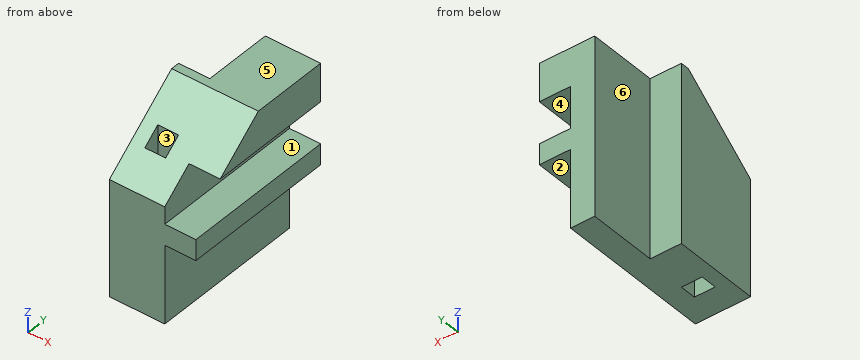
Solid Edge part; units mm, degrees
sketch "Sketch1" plane through (0, 0, 0) normal (0, 0, 1) x (1, 0, 0)
  line L0 (25, -45) -> (25, 45)
  line L1 (25, 45) -> (-25, 45)
  line L2 (-25, 45) -> (-25, -45)
  line L3 (-25, -45) -> (25, -45)
extrude "Protrusion1" add sketch "Sketch1" along normal blind 103
sketch "Sketch2" plane through (0, -45, 51.5) normal (0, -1, 0) x (1, 0, 0)
  line L0 (25, 5.5) -> (25, 29.5)
  line L1 (25, 29.5) -> (7, 29.5)
  line L2 (7, 29.5) -> (7, 5.5)
  line L3 (7, 5.5) -> (25, 5.5)
  line L4 (25, -6.5) -> (25, -51.5)
  line L5 (25, -51.5) -> (7, -51.5)
  line L6 (7, -51.5) -> (7, -6.5)
  line L7 (7, -6.5) -> (25, -6.5)
extrude "Cutout1" cut sketch "Sketch2" against normal up to next
sketch "Sketch3" plane through (-25, 0, 51.5) normal (-1, 0, 0) x (0, -1, 0)
  line L0 (0, 51.5) -> (45, 15.5)
extrude "Cutout2" cut sketch "Sketch3" against normal up to next material side at (-25, -22.5312, 85.039)
sketch "Sketch4" plane through (0, 22.5, 103) normal (0, 0, 1) x (1, 0, 0)
  line L0 (-7, -17.5) -> (-7, 22.5)
  line L1 (-7, 22.5) -> (-25, 22.5)
  line L2 (-25, 22.5) -> (-25, -17.5)
  line L3 (-25, -17.5) -> (-7, -17.5)
extrude "Cutout3" cut sketch "Sketch4" against normal up to next
sketch "Sketch5" plane through (0, 0, 0) normal (0, 0, 1) x (1, 0, 0)
  line L0 (-17, -29.3826) -> (-5, -29.3826)
  line L1 (-5, -29.3826) -> (-5, -20.0122)
  line L2 (-5, -20.0122) -> (-17, -20.0122)
  line L3 (-17, -20.0122) -> (-17, -29.3826)
extrude "Cutout4" cut sketch "Sketch5" along normal up to next
Here's how the part is built. I have some questions about the finished solid (model axes, mm). Face numbers are marked on the shaded views. A direction names the side the tool comes from. Round coordinates to 2 decimals unless told otherwise and drop trailing zeros. Order: outer loops, then holes, each group sorted by start corner. A loop starts at its lowest first (then second) coordinate and runs counter-clockwise, first axis right, second up. Notation, with made-up numbers: (85, 33.25) -> (102, 33.25) arc R25 cw to (102, 62.25) -> close; hole circle Ø8 at (-10, -20.75). An arc over 180 degrees is marked (long way). Use CSV: the item, a comma, the result in double quotes.
1. I want a section at B-B on z = 8. List the corners of the cut face in (x, y) for me.
Recorded:
outline,"(-25, -45) -> (7, -45) -> (7, 45) -> (-7, 45) -> (-7, 5) -> (-25, 5) -> close; hole (-17, -29.38) -> (-5, -29.38) -> (-5, -20.01) -> (-17, -20.01) -> close"
2. I'm going to push flat-ended pins straight in: P1, Ø4, axis at x = -5.5, y = -20.5, coming from the +Z side; P2, Ø6, axis at x = 8, y = -19.5, coming from the +Z side; P3, Ø7, axis at y = 9.5, z = 65.5, coming from the +X side; P4, Ø12, axis at x = -17.5, y = 34.5, coming from the +Z side. Where does each tip first touch, or does it pass through?
Recorded:
P1,"stops at z = 88.2"
P2,"stops at z = 89.8"
P3,"stops at x = 7"
P4,"passes through"
3. Thinking about a two-plate mould opening in Z: for the marked faces 4, 5 and 6, which applies, pulls with the +Z half, pulls with the -Z half, needs draft (parallel to the pull), parting line crosses it, or undercut?
Recorded:
face 4,"undercut"
face 5,"pulls with the +Z half"
face 6,"needs draft"
4. I need wall thicknesses on line 1 along Z through (x, y) = (16, 23); line 2 along X through (y, z) = (-22, 19.5); line 3 along Y through (x, z) = (-9.5, 27.5). Which ranges of each line are inside material? Lowest first, please.
Recorded:
line 1,"z = 45 to 57, 81 to 103"
line 2,"x = -25 to -17, -5 to 7"
line 3,"y = -45 to -29.38, -20.01 to 5"
5. Which directions (+Z, -Z, +X, -X, +Y, -Y) give clear straight access to the entire face, cutting with the end or side of a thin tool? Please do the marked faces 1, 2 and 3.
Recorded:
face 1,"+X, +Y, -Y"
face 2,"-Z, +X, +Y, -Y"
face 3,"+Z, -Z"
6. I want a section at A-A on x = -12. List the corners of the cut face in (y, z) for me, and give its area (3 significant figures).
Recorded:
outline,"(-45, 0) -> (-29.38, 0) -> (-29.38, 79.49) -> (-45, 67) -> close; (-20.01, 0) -> (5, 0) -> (5, 103) -> (0, 103) -> (-20.01, 86.99) -> close"
area,"3,560 mm2"
7. I want a section at C-C on y = -24. List the corners of the cut face in (x, z) for me, and give its area (3 significant figures).
Recorded:
outline,"(-25, 0) -> (-17, 0) -> (-17, 83.8) -> (-25, 83.8) -> close; (-5, 0) -> (7, 0) -> (7, 45) -> (25, 45) -> (25, 57) -> (7, 57) -> (7, 81) -> (25, 81) -> (25, 83.8) -> (-5, 83.8) -> close"
area,"1,940 mm2"
8. I want a section at D-D on y = 22.5. List the corners of the cut face in (x, z) for me.
Recorded:
outline,"(-7, 0) -> (7, 0) -> (7, 45) -> (25, 45) -> (25, 57) -> (7, 57) -> (7, 81) -> (25, 81) -> (25, 103) -> (-7, 103) -> close"
